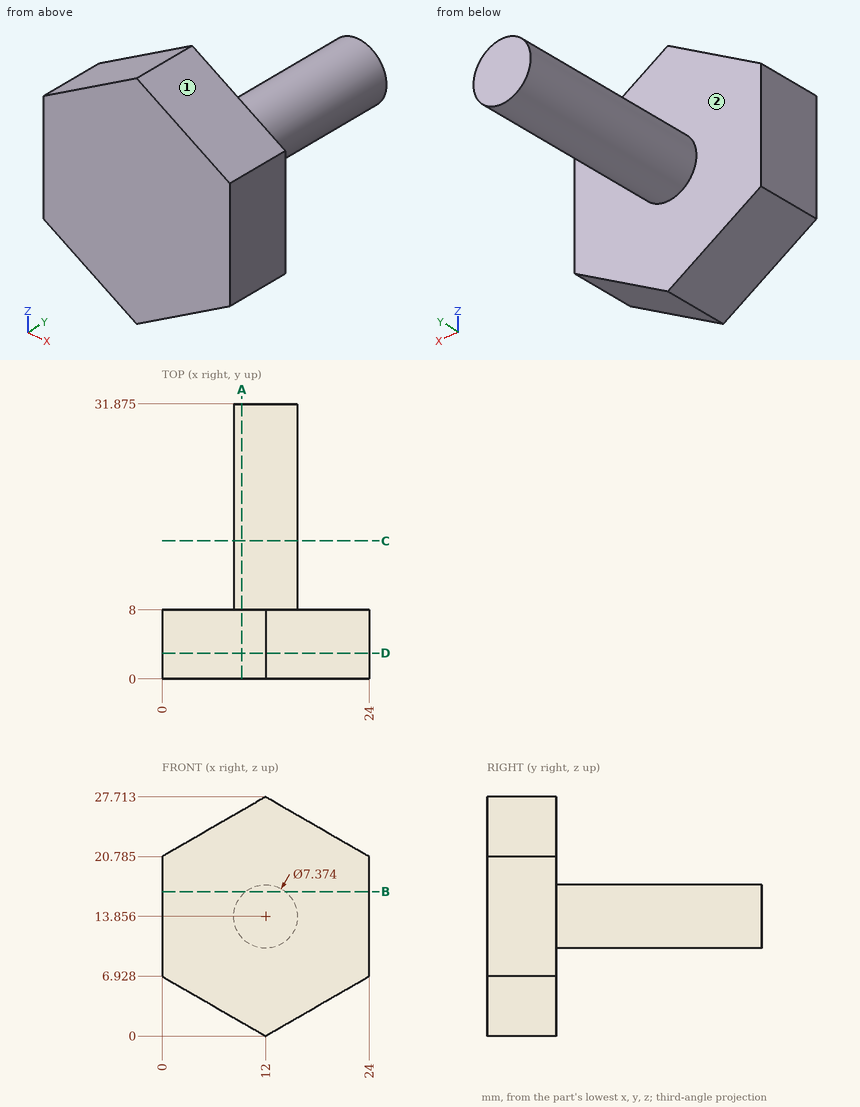
Drawing for the job (mm, zero at the part's lowest x, y, z). A direction names the side the tool comes from. Give positions to 0.01 mm unless a question says otherwise; leave off trailing zeros. Order: outer loops, then holes, each group sorted by start corner. A loop starts at its lowest first (then second) coordinate and runs counter-clockwise, first axis right, second up. Notation, with made-up numbers: (-33, 84.25) - (13, 84.25) arc R26 ccw to (13, 120.25) - close; hole circle Ø3 at (-5, -28). An arc over 180 degrees is marked (long way). Write item = value, one per line. Start each with the question number.
1. Cut at C-C, the plane y = 16. List the corners of the cut face in (x, z).
2. Drop flat-ended pins along their axis: P1, Ø4, axis at x = 6.5, z = 6, coming from the -Y side; P2, Ø5, axis at x = 15.5, z = 24.5, coming from the +Y side; P3, Ø12, axis at y = 15, z = 19.5, coming from the -X side; P4, Ø2, axis at x = 8, y = 16, coming from the -Z side (1 decimal). Give the stop position or say it passes through.
3. Which spindle directions (+Z, -Z, +X, -X, +Y, -Y) get a long thin tool onto all of the face, cutting with end or side? Do the marked faces 1 and 2. Say none if no direction does.
4. Probe line 1 along Y through (x, z) = (17, 5.5); line 2 along Z through (x, y) = (10, 15.5) (1 decimal); line 3 along Z through (x, y) = (12.75, 18) (1 decimal). List the from-to ranges inside material, lowest first.
5. Cut at A-A, the plane x = 9.25. List the corners of the cut face in (y, z) (1 decimal).
6. Cut at D-D, the plane y = 3. List the corners of the cut face in (x, z) (1 decimal).
7. Cut at B-B, the plane z = 16.75. List the corners of the cut face in (x, y) (1 decimal).
Taken from the geometry:
q1.outline = circle Ø7.37 at (12, 13.86)
q2.P1 = 0
q2.P2 = 8
q2.P3 = 8.31
q2.P4 = 11.7
q3.face_1 = +Z, +X, +Y, -Y
q3.face_2 = +Y
q4.line_1 = 0 to 8
q4.line_2 = 10.8 to 17
q4.line_3 = 10.2 to 17.5
q5.outline = (0, 1.6) - (8, 1.6) - (8, 11.4) - (31.9, 11.4) - (31.9, 16.3) - (8, 16.3) - (8, 26.1) - (0, 26.1) - close
q6.outline = (0, 6.9) - (12, 0) - (24, 6.9) - (24, 20.8) - (12, 27.7) - (0, 20.8) - close
q7.outline = (0, 0) - (24, 0) - (24, 8) - (14.3, 8) - (14.3, 31.9) - (9.7, 31.9) - (9.7, 8) - (0, 8) - close
